from build123d import *

# Parameters (mm, degrees)
SKETCH1_W           = 23.495
SKETCH1_H           = 22.86
BOSS_EXTRUDE1_DEPTH = 1.6002
SKETCH2_W           = 4.064
SKETCH2_H           = 5.08
BOSS_EXTRUDE2_DEPTH = 1.7018
FILLET1_R           = 2.54
SKETCH4_R           = 1.778
CUT_EXTRUDE1_DEPTH  = 2.6002


with BuildPart() as part:
    # Sketch1 → Boss-Extrude1 (new body)
    with BuildSketch(Plane(origin=(0, 0, 0), x_dir=(1, 0, 0), z_dir=(0, 1, 0))):
        Rectangle(SKETCH1_W, SKETCH1_H)
    extrude(amount=BOSS_EXTRUDE1_DEPTH)

    # Sketch2 → Boss-Extrude2 (add)
    with BuildSketch(Plane(origin=(0, 1.6002, 0), x_dir=(1, 0, 0), z_dir=(0, 1, 0))):
        Rectangle(SKETCH2_W, SKETCH2_H)
    extrude(amount=BOSS_EXTRUDE2_DEPTH)

    # Fillet1
    fillet1_edges = [part.edges().sort_by_distance(p)[0] for p in [
        (11.7475, 0.8001, 11.43),
        (-11.7475, 0.8001, 11.43),
        (-11.7475, 0.8001, -11.43),
        (11.7475, 0.8001, -11.43),
    ]]
    fillet(fillet1_edges, radius=FILLET1_R)

    # Sketch4 → Cut-Extrude1 (cut, through all)
    with BuildSketch(Plane(origin=(0, 1.6002, 0), x_dir=(1, 0, 0), z_dir=(0, 1, 0))):
        with Locations((-8.1915, -7.874)):
            Circle(SKETCH4_R)
        with Locations((-8.1915, 7.874)):
            Circle(SKETCH4_R)
        with Locations((8.1915, 7.874)):
            Circle(SKETCH4_R)
        with Locations((8.1915, -7.874)):
            Circle(SKETCH4_R)
    extrude(amount=-CUT_EXTRUDE1_DEPTH, mode=Mode.SUBTRACT)


solid = part.part
Could you check a few things on this model? Use its own coordinates, in mm. A direction names the side the tool comes from. Give positions to 0.01 mm unless a question says otherwise; leave off trailing zeros. Order: outer loops, then holes, each group sorted by start corner. A loop starts at its lowest first (then second) coordinate and runs counter-clockwise, first axis right, second up.
1. I need wall thicknesses on L1, parallel to X at y = 0.45, z = 8.75; L2, parallel to X at y = 0.6, z = -9.25; L3, parallel to Y at x = 7.75, z = 1.25. Which ranges of each line are inside material? Lowest first, please.
Answers below:
L1: x = -11.75 to -9.74, -6.64 to 6.64, 9.74 to 11.75
L2: x = -11.72 to -9.32, -7.07 to 7.07, 9.32 to 11.72
L3: y = 0 to 1.6
2. Suppose I cut it at D-D (x = -1.75). Write out the boundary of the cut face in (y, z).
Answers below:
outline: (0, -11.43) - (1.6, -11.43) - (1.6, -2.54) - (3.3, -2.54) - (3.3, 2.54) - (1.6, 2.54) - (1.6, 11.43) - (0, 11.43) - close
3. Suppose I cut it at A-A (y = 0.75). Write out the boundary of the cut face in (x, z), plus the area to 3 significant figures.
Answers below:
outline: (-11.75, -8.89) arc R2.54 ccw to (-9.21, -11.43) - (9.21, -11.43) arc R2.54 ccw to (11.75, -8.89) - (11.75, 8.89) arc R2.54 ccw to (9.21, 11.43) - (-9.21, 11.43) arc R2.54 ccw to (-11.75, 8.89) - close; hole circle Ø3.56 at (-8.19, -7.87); hole circle Ø3.56 at (-8.19, 7.87); hole circle Ø3.56 at (8.19, -7.87); hole circle Ø3.56 at (8.19, 7.87)
area: 492 mm2
4. Thinking about a two-plate mould opening in X: for faces 3 (the flat face through (0, 2, -2.54)), 4 (the cylindrical face through (-6.496, 0.811, -8.408)), 5 (the flat face through (-2.032, 2, 0)), which applies, +X half, -X half, draft (parallel to the pull), parting line (faces both ways), or undercut?
Answers below:
face 3: draft
face 4: undercut
face 5: -X half
5. For pin 1 (5 mm diameter, centred on x = 7.5, z = 0.5, fed in from +Y); pin 2 (0.5 mm diameter, centred on y = 2.5, z = -0.5, fed in from +X); pin 3 (0.5 mm diameter, centred on x = 0.5, y = 2, fed in from -Z); pin 4 (3 mm diameter, centred on x = -8.19, z = 7.87, fed in from -Y) (3 decimals), each with a flat end and sliding along its axis, tell me the tip position at first contact or that it passes through.
Answers below:
pin 1: stops at y = 1.6
pin 2: stops at x = 2.03
pin 3: stops at z = -2.54
pin 4: passes through
6. Which directions (+Z, -Z, +X, -X, +Y, -Y) give clear straight access to the entire face, cutting with the end or side of a thin tool? Please do faces 1 (the cylindrical face through (-11.02, 0.81, -10.67)), 2 (the flat face through (2.032, 2, 0)).
Answers below:
face 1: -Z, -X, +Y, -Y
face 2: +Z, -Z, +X, +Y
7. Suppose I cut it at C-C (z = -1.25). Write out the boundary of the cut face in (x, y), plus the area to 3 significant figures.
Answers below:
outline: (-11.75, 0) - (11.75, 0) - (11.75, 1.6) - (2.03, 1.6) - (2.03, 3.3) - (-2.03, 3.3) - (-2.03, 1.6) - (-11.75, 1.6) - close
area: 44.5 mm2
8. Suppose I cut it at B-B (x = 6.75). Write out the boundary of the cut face in (y, z), plus the area to 3 significant figures.
Answers below:
outline: (0, -11.43) - (1.6, -11.43) - (1.6, -8.91) - (0, -8.91) - close; (0, -6.83) - (1.6, -6.83) - (1.6, 6.83) - (0, 6.83) - close; (0, 8.91) - (1.6, 8.91) - (1.6, 11.43) - (0, 11.43) - close
area: 29.9 mm2
